Can you work these out from the model? Positions are in its coordinate system, mm. Round coordinates to 2 decimals unless told otherwise and drop trailing zeros.
from build123d import *

# Parameters (mm, degrees)
PAD_DEPTH           = 10
HOLE004_D           = 5.5
HOLE004_DEPTH       = 25
HOLE004_CBORE_D     = 10
HOLE004_CBORE_DEPTH = 4
SKETCH010_R         = 2.9
HOLE005_DEPTH       = 25


with BuildPart() as part:
    # Sketch → Pad (new body)
    with BuildSketch(Plane.XY):
        Polygon((0, 70), (300, 70), (310, 60), (310, -60), (300, -70), (0, -70), (-10, -45), (-40, -45), (-40, 45), (-10, 45), align=None)
    extrude(amount=PAD_DEPTH)

    # Hole004
    with Locations(Plane.XY.offset(10)):
        with Locations((-15, 0), (65, 0), (140, 0), (227.5, 0)):
            CounterBoreHole(HOLE004_D / 2, HOLE004_CBORE_D / 2, HOLE004_CBORE_DEPTH, depth=HOLE004_DEPTH)

    # Sketch010 (on Face4 of Hole004) → Hole005 (cut)
    with BuildSketch(Plane(origin=(0, 0, 0), x_dir=(1, 0, 0), z_dir=(0, 0, -1))):
        with Locations((25, 60)):
            Circle(SKETCH010_R)
        with Locations((100, 60)):
            Circle(SKETCH010_R)
        with Locations((200, 60)):
            Circle(SKETCH010_R)
        with Locations((285, 60)):
            Circle(SKETCH010_R)
        with Locations((25, -60)):
            Circle(SKETCH010_R)
        with Locations((100, -60)):
            Circle(SKETCH010_R)
        with Locations((200, -60)):
            Circle(SKETCH010_R)
        with Locations((285, -60)):
            Circle(SKETCH010_R)
    extrude(amount=-HOLE005_DEPTH, mode=Mode.SUBTRACT)


solid = part.part
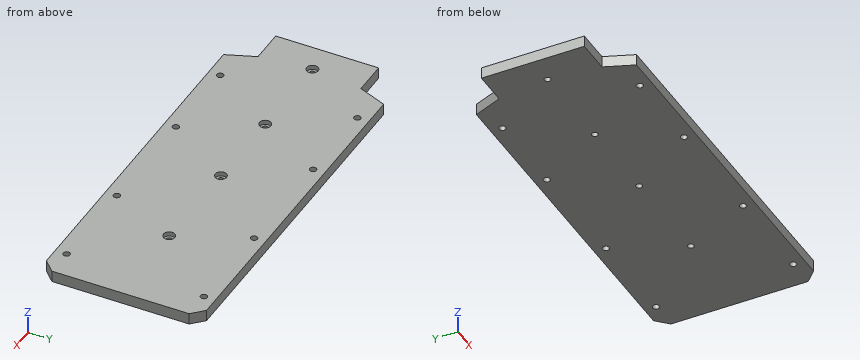
(1) Please list where these lines run through material, in increasing order: probe 1 along Y at (x, z) = (25, 3.25); probe 2 along X at (y, z) = (-1.5, 5.75); probe 3 along X at (y, z) = (60, 7).
(2) I want a section at A-A, the plane z = 4. Give the number of separate pieces and of enclosed holes in the cut face, plus the area to 3 significant figures.
(3) I'm going to push flat-ended pins straight in: pin 1 Ø4.5 at (x, y) = (140, 0) entering from +Z; pin 2 Ø5 at (x, y) = (66.5, 0.5) entering from +Z. Where does each tip first touch, or does it pass through?
Ans:
1. probe 1: y = -70 to -62.9, -57.1 to 57.1, 62.9 to 70
1. probe 2: x = -40 to -17.3, -12.7 to 62.7, 67.3 to 137.7, 142.3 to 225.2, 229.8 to 310
1. probe 3: x = -4 to 22.1, 27.9 to 97.1, 102.9 to 197.1, 202.9 to 282.1, 287.9 to 310
2. separate pieces: 1
2. enclosed holes: 12
2. area: 46,800 mm2
3. pin 1: passes through
3. pin 2: stops at z = 6
